from build123d import *

# Parameters (mm, degrees)
EXTRUDE_1079_DEPTH     = 8
FILLET_4_R             = 3
FILLET_5_R             = 2
SKETCH_13_W            = 3
SKETCH_13_H            = 8
SKETCH_13_H_2          = 2
CUT_EXTRUDE_2700_DEPTH = 1
HOLE_WIZARD_M2_D       = 1.6
FILLET_6_R             = 3
FILLET_7_R             = 5
SKETCH_19_W            = 4
SKETCH_19_H            = 18
CUT_EXTRUDE_4512_DEPTH = 62.155364655
CUT_EXTRUDE_1_REACH    = 71.276
SKETCH_20_R            = 2.5
SKETCH_20_R_2          = 1.5
CUT_EXTRUDE_2_DEPTH    = 62.155364655
FILLET_8_R             = 1.5


with BuildPart() as part:
    # Эскиз8 → Extrude 1079 (new body)
    with BuildSketch(Plane.XY):
        Polygon((0, -18.75), (0, 18.75), (15, 18.75), (35, -1.25), (35, -53.75), align=None)
        Polygon((32, -46.507359313), (3, -17.507359313), (3, 15.75), (13.757359313, 15.75), (32, -2.492640687), align=None, mode=Mode.SUBTRACT)
    extrude(amount=-EXTRUDE_1079_DEPTH)

    # Скругление4
    fillet_4_edges = [part.edges().sort_by_distance(p)[0] for p in [
        (3, -17.507359313, -4),
        (3, 15.75, -4),
        (15, 18.75, -4),
        (35, -1.25, -4),
        (0, -18.75, -4),
        (0, 18.75, -4),
    ]]
    fillet(fillet_4_edges, radius=FILLET_4_R)

    # Скругление5
    fillet_5_edges = [part.edges().sort_by_distance(p)[0] for p in [
        (13.757359313, 15.75, -4),
        (32, -46.507359313, -4),
    ]]
    fillet(fillet_5_edges, radius=FILLET_5_R)

    # Эскиз13 → Cut-Extrude 2700 (cut)
    with BuildSketch(Plane(origin=(0, 0, 0), x_dir=(-1, 0, 0), z_dir=(0, 0, -1))):
        with Locations((-1.5, 0)):
            Rectangle(SKETCH_13_W, SKETCH_13_H)
        with Locations((-33.5, -26)):
            Rectangle(SKETCH_13_W, SKETCH_13_H_2)
    extrude(amount=CUT_EXTRUDE_2700_DEPTH, mode=Mode.SUBTRACT)

    # Крепление рамки M2 (through all)
    with Locations(Plane.XY):
        with Locations((2, -18.3), (3, 16.07), (32, -46.75), (33, -2.17)):
            Hole(HOLE_WIZARD_M2_D / 2)

    # Скругление6
    fillet_6_edges = [part.edges().sort_by_distance(p)[0] for p in [
        (35, -53.75, -4),
    ]]
    fillet(fillet_6_edges, radius=FILLET_6_R)

    # Скругление7
    fillet_7_edges = [part.edges().sort_by_distance(p)[0] for p in [
        (32, -2.492640687, -4),
    ]]
    fillet(fillet_7_edges, radius=FILLET_7_R)

    # Эскиз19 → Cut-Extrude 4512 (cut, through all)
    with BuildSketch(Plane.XY):
        with Locations((33, -14.38)):
            Rectangle(SKETCH_19_W, SKETCH_19_H)
    extrude(amount=-CUT_EXTRUDE_4512_DEPTH, mode=Mode.SUBTRACT)

    # Эскиз20 → Вырез-Вытянуть1 (cut, up to next)
    with BuildSketch(Plane(origin=(16.875, 16.875, 0), x_dir=(0, 0, -1), z_dir=(0.7071067811865488, 0.7071067811865462, 0)), mode=Mode.PRIVATE) as cut_extrude_1_sk1:
        with Locations(Location((4, -7.570990258, 0), (0, 0, 90))):
            Circle(SKETCH_20_R)
    cut_extrude_1_tool1 = extrude(cut_extrude_1_sk1.sketch, amount=-CUT_EXTRUDE_1_REACH, mode=Mode.PRIVATE) & part.part
    # Эскиз20 → Вырез-Вытянуть1 (cut, up to next)
    with BuildSketch(Plane(origin=(16.875, 16.875, 0), x_dir=(0, 0, -1), z_dir=(0.7071067811865488, 0.7071067811865462, 0)), mode=Mode.PRIVATE) as cut_extrude_1_sk2:
        with Locations(Location((4.0519, -17.407536383, 0), (0, 0, 90))):
            Circle(SKETCH_20_R_2)
    cut_extrude_1_tool2 = extrude(cut_extrude_1_sk2.sketch, amount=-CUT_EXTRUDE_1_REACH, mode=Mode.PRIVATE) & part.part
    add(cut_extrude_1_tool1.solids().sort_by_distance((22.228499, 11.521501, -4))[0], mode=Mode.SUBTRACT)
    add(cut_extrude_1_tool2.solids().sort_by_distance((29.183987, 4.566013, -4.0519))[0], mode=Mode.SUBTRACT)

    # Эскиз21 → Вырез-Вытянуть2 (cut, through all)
    with BuildSketch(Plane.XY):
        Polygon((26.355559895, 7.394440105), (25.294899724, 6.333779933), (30.951753973, 0.676925683), (32.012414145, 1.737585855), align=None)
    extrude(amount=-CUT_EXTRUDE_2_DEPTH, mode=Mode.SUBTRACT)

    # Скругление8
    fillet_8_edges = [part.edges().sort_by_distance(p)[0] for p in [
        (30.951753973, 0.676925683, -4),
        (25.294899724, 6.333779933, -4),
    ]]
    fillet(fillet_8_edges, radius=FILLET_8_R - 0.0001)  # a hair under: the kernel refuses the full size


solid = part.part
Build history of the part. All positions in model axes, mm. A direction names the side the tool comes from. Round coordinates to 2 decimals unless told otherwise and drop trailing zeros. Loops run counter-clockwise (first coordinate to the right, second up) from the corner with the lowest first, then second, coordinate; pieces in that order, holes last. Notation, with made-up numbers: (-30, -33) -> (25, -33) arc R26 cw to (25, 0) -> close; hole circle Ø9 at (24.25, 18). An arc over 180 degrees is marked (long way). One line per item, written item: value. Start each with the question number.
Q1. Two-plate mould, pull along Y, no slides. Class faces 1 (the face through (0.22, -18.64, -4.06)), 2 (the face through (31.237, -46.51, -4.056)), 3 (the face through (31, 1.3, -4.1)): released by +Y, released by -Y, zero draft, split by the parting line, or undercut.
Q2. Cut at A-A on y = -30. List the corners of the cut face in (x, z), plus the area to 3 significant figures.
Q3. Drop flat-ended pins along their axis: pin 1 Ø0.9 at (x, y) = (1.5, 0.5) entering from +Z; pin 2 Ø3 at (y, z) = (-19.5, -2) entering from +X; pin 3 Ø2 at (x, z) = (27.5, -3) entering from +Y; pin 4 Ø1.3 at (x, y) = (33, -2.17) entering from -Z. Give the stop position or say it passes through.
Q4. Probe line 1 along Y through (x, z) = (33, -2.75); line 2 along X through (y, z) = (10, -1); line 3 along Y through (x, z) = (20, -1). List the from-to ranges inside material, lowest first.
Q5. 3-axis set-ups, long thin cutter, end or side, ignore diameter. For faces 4 (the face through (33, -23.38, -4)), 5 (the face through (3, -2, -4)), 6 (the face through (21.41, 10.25, -1.52)): which of +Z, -Z, +X, -X, +Y, -Y reach the whole face in a straight line?
Q6. Cut at B-B on x = 5. List the corners of the cut face in (y, z).
Computed:
1. face 1: released by -Y
1. face 2: undercut
1. face 3: released by +Y
2. outline: (11.25, -8) -> (15.49, -8) -> (15.49, 0) -> (11.25, 0) -> close; (32, -8) -> (35, -8) -> (35, 0) -> (32, 0) -> close
2. area: 57.9 mm²
3. pin 1: z = -1
3. pin 2: x = 6.49
3. pin 3: y = 5.13
3. pin 4: through
4. line 1: -49.34 to -23.38, -5.38 to -2.97, -1.37 to 0.75
4. line 2: 0 to 3, 19.51 to 23.75
4. line 3: -38.75 to -34.51, 9.51 to 13.75
5. face 4: +Z, -Z, +X
5. face 5: +Z, -Z
5. face 6: none
6. outline: (-23.75, -8) -> (-19.51, -8) -> (-19.51, 0) -> (-23.75, 0) -> close; (15.58, -8) -> (18.75, -8) -> (18.75, 0) -> (15.58, 0) -> close
